```python
from build123d import *

# Parameters (mm, degrees)
F0_R      = 46.570843
F1_DEPTH  = 25.4
F2_R      = 13.732037
F3_DEPTH  = 25.4
F4_R      = 12.7
F5_DEPTH  = 25.4
F5_FACE_R = 12.7
F6_DEPTH  = 25.4
F7_R      = 12.7
F8_DEPTH  = 25.4


with BuildPart() as f1:
    # F0 (on Top) → F1 (new body)
    with BuildSketch(Plane.XY):
        Circle(F0_R)
    extrude(amount=F1_DEPTH)

    # F2 (on Top) → F3 (join)
    with BuildSketch(Plane.XY):
        Circle(F2_R)
    extrude(amount=F3_DEPTH)

    # F4 (on face) → F5 (join)
    with BuildSketch(Plane.XY.offset(25.4)):
        Circle(F4_R)
    extrude(amount=F5_DEPTH)

    # F5_face (on face) → F6 (cut)
    with BuildSketch(Plane.XY.offset(50.8)):
        Circle(F5_FACE_R)
    extrude(amount=-F6_DEPTH, mode=Mode.SUBTRACT)

    # F7 (on face) → F8 (cut)
    with BuildSketch(Plane.XY.offset(25.4)):
        Circle(F7_R)
    extrude(amount=-F8_DEPTH, mode=Mode.SUBTRACT)


solid = f1.part
```
Build history of the part. All positions in model axes, mm. Give positions to 0.01 mm unless a question says otherwise; leave off trailing zeros. Order: outer loops, then holes, each group sorted by start corner. A loop starts at its lowest first (then second) coordinate and runs counter-clockwise, first axis right, second up. Notation, with made-up numbers: M 53.25,82 L 95.25,82 A27 cw 95.25,120 Z; hole C 74.5,4 d3. An arc over 180 degrees is marked long. Write item = value, one per line. Start each with the question number.
(1) Slice it at A-A on x = 0. Write the cut outline in (y, z), plus the area to 3 significant figures.
(2) Pin check, flat tips, straight feed: pin 1 Ø1 at (x, z) = (-22, 12) entering from +Y; pin 2 Ø12 at (x, y) = (33, 3.5) entering from -Z; pin 3 Ø3 at (y, z) = (33.5, 9.5) entering from -X; pin 4 Ø12 at (x, z) = (5.5, 21.5) entering from -Y. Stop position of each tip, or through.
(3) Slice it at C-C on z = 20. Write the cut outline in (x, y).
(4) Probe L1, parallel to Y at x = 0, z = 12.5; L2, parallel to Y at x = 9.5, z = 1.5; L3, parallel to X at y = -18, z = 14. List the from-to ranges inside material, lowest first. Write a range as [from, to].
(5) Two-plate mould, pull along Y, no slides. Class faces 1 (the cylindrical face through (-2.75, -12.4, 12.88)), 2 (the flat face through (10, -10, 0)), 3 (the cylindrical face through (-34.3, 31.5, 12.5)): released by +Y, released by -Y, zero draft, split by the parting line, or undercut.
(6) Slice it at D-D on x = -30. Write the cut outline in (y, z), plus the area to 3 significant figures.
Responses:
q1.outline = M -46.57,0 L -12.7,0 L -12.7,25.4 L -46.57,25.4 Z; M 12.7,0 L 46.57,0 L 46.57,25.4 L 12.7,25.4 Z
q1.area = 1,720 mm2
q2.pin_1 = 41.31
q2.pin_2 = 0
q2.pin_3 = -33.84
q2.pin_4 = -46.57
q3.outline = C 0,0 d93.14; hole C 0,0 d25.4
q4.L1 = [-46.57, -12.7], [12.7, 46.57]
q4.L2 = [-45.59, -8.43], [8.43, 45.59]
q4.L3 = [-42.95, 42.95]
q5.face_1 = undercut
q5.face_2 = zero draft
q5.face_3 = split by the parting line
q6.outline = M -35.62,0 L 35.62,0 L 35.62,25.4 L -35.62,25.4 Z
q6.area = 1,810 mm2
